```python
from build123d import *

# Parameters (mm, degrees)
CROQUIS1_W                   = 482.6
CROQUIS1_H                   = 634.238
BRIDA_BASE1_DEPTH            = 1.524
CROQUIS6_R                   = 3.9624
CROQUIS6_W                   = 6.35
CROQUIS6_H                   = 3.048
CORTAR_EXTRUIR1_DEPTH        = 399.487732229
BRIDA_START                  = -218.948
BRIDA_DE_ARISTA1_DEPTH       = 437.896
BRIDA_START_2                = -219.1004
BRIDA_DE_ARISTA1_2_OUTLINE_W = 0.1524
BRIDA_DE_ARISTA1_2_OUTLINE_H = 1.524
BRIDA_DE_ARISTA1_2_DEPTH     = 0.1524
BRIDA_START_3                = 218.948
BRIDA_DE_ARISTA1_3_OUTLINE_W = 0.1524
BRIDA_DE_ARISTA1_3_OUTLINE_H = 1.524
BRIDA_DE_ARISTA1_3_DEPTH     = 0.1524
BRIDA_DE_ARISTA1_4_DEPTH     = 437.896
CORTAR_EXTRUIR2_REACH        = 400.806
CROQUIS13_R                  = 3.9624
CROQUIS13_R_2                = 2.8956
CROQUIS13_R_3                = 1.27
CROQUIS13_W                  = 139.7
CROQUIS13_H                  = 124.714


# Read off the part's stored shape, not the designer's step: Brida de arista1
# Sheet-metal steps are written as plain solids
with BuildPart() as part:
    # Croquis1 → Brida base1 (new body)
    with BuildSketch(Plane.XY):
        Rectangle(CROQUIS1_W, CROQUIS1_H)
    extrude(amount=-BRIDA_BASE1_DEPTH)

    # Croquis6 → Cortar-Extruir1 (cut, through all)
    with BuildSketch(Plane.XY):
        with Locations((231.648, 317.627)):
            Circle(CROQUIS6_R)
        with Locations((-231.648, 317.627)):
            Circle(CROQUIS6_R)
        with Locations((-231.648, -317.627)):
            Circle(CROQUIS6_R)
        with Locations((231.648, -317.627)):
            Circle(CROQUIS6_R)
        with Locations((-222.123, 315.595)):
            Rectangle(CROQUIS6_W, CROQUIS6_H)
        with Locations((222.123, 315.595)):
            Rectangle(CROQUIS6_W, CROQUIS6_H)
        with Locations((-222.123, -315.595)):
            Rectangle(CROQUIS6_W, CROQUIS6_H)
        with Locations((222.123, -315.595)):
            Rectangle(CROQUIS6_W, CROQUIS6_H)
    extrude(amount=-CORTAR_EXTRUIR1_DEPTH, mode=Mode.SUBTRACT)

    # Brida de arista1 outline → Brida de arista1 (cut)
    with BuildSketch(Plane.YZ.offset(BRIDA_START)):
        with BuildLine():
            ThreePointArc((-316.710645431, -1.524), (-315.595, -0.408354569), (-314.071, 0))
            Line((-314.071, 0), (-317.119, 0))
            Line((-317.119, 0), (-317.119, -1.524))
            Line((-317.119, -1.524), (-316.710645431, -1.524))
        make_face()
        with BuildLine():
            Line((317.119, 0), (314.071, 0))
            ThreePointArc((314.071, 0), (315.595, -0.408354569), (316.710645431, -1.524))
            Line((316.710645431, -1.524), (317.119, -1.524))
            Line((317.119, -1.524), (317.119, 0))
        make_face()
    extrude(amount=BRIDA_DE_ARISTA1_DEPTH, mode=Mode.SUBTRACT)

    # Brida de arista1 2 outline → Brida de arista1 2 (cut)
    with BuildSketch(Plane.YZ.offset(BRIDA_START_2)):
        with Locations((-313.9948, -0.762)):
            Rectangle(BRIDA_DE_ARISTA1_2_OUTLINE_W, BRIDA_DE_ARISTA1_2_OUTLINE_H)
        with Locations((313.9948, -0.762)):
            Rectangle(BRIDA_DE_ARISTA1_2_OUTLINE_W, BRIDA_DE_ARISTA1_2_OUTLINE_H)
    extrude(amount=BRIDA_DE_ARISTA1_2_DEPTH, mode=Mode.SUBTRACT)

    # Brida de arista1 3 outline → Brida de arista1 3 (cut)
    with BuildSketch(Plane.YZ.offset(BRIDA_START_3)):
        with Locations((-313.9948, -0.762)):
            Rectangle(BRIDA_DE_ARISTA1_3_OUTLINE_W, BRIDA_DE_ARISTA1_3_OUTLINE_H)
        with Locations((313.9948, -0.762)):
            Rectangle(BRIDA_DE_ARISTA1_3_OUTLINE_W, BRIDA_DE_ARISTA1_3_OUTLINE_H)
    extrude(amount=BRIDA_DE_ARISTA1_3_DEPTH, mode=Mode.SUBTRACT)

    # Brida de arista1 4 outline → Brida de arista1 4 (add)
    with BuildSketch(Plane.YZ.offset(BRIDA_START)):
        with BuildLine():
            ThreePointArc((-315.595, -3.048), (-315.148630735, -1.970369265), (-314.071, -1.524))
            Line((-314.071, -1.524), (-316.710645431, -1.524))
            ThreePointArc((-316.710645431, -1.524), (-317.015141918, -2.259119551), (-317.119, -3.048))
            Line((-317.119, -3.048), (-317.119, -16.002))
            Line((-317.119, -16.002), (-315.595, -16.002))
            Line((-315.595, -16.002), (-315.595, -3.048))
        make_face()
        with BuildLine():
            Line((316.710645431, -1.524), (314.071, -1.524))
            ThreePointArc((314.071, -1.524), (315.148630735, -1.970369265), (315.595, -3.048))
            Line((315.595, -3.048), (315.595, -16.002))
            Line((315.595, -16.002), (317.119, -16.002))
            Line((317.119, -16.002), (317.119, -3.048))
            ThreePointArc((317.119, -3.048), (317.015141918, -2.259119551), (316.710645431, -1.524))
        make_face()
    extrude(amount=BRIDA_DE_ARISTA1_4_DEPTH)

    # Croquis13 → Cortar-Extruir2 (cut, up to next)
    with BuildSketch(Plane.XY, mode=Mode.PRIVATE) as cortar_extruir2_sk1:
        with Locations((-231.648, -158.877)):
            Circle(CROQUIS13_R)
    cortar_extruir2_tool1 = extrude(cortar_extruir2_sk1.sketch, amount=-CORTAR_EXTRUIR2_REACH, mode=Mode.PRIVATE) & part.part
    # Croquis13 → Cortar-Extruir2 (cut, up to next)
    with BuildSketch(Plane.XY, mode=Mode.PRIVATE) as cortar_extruir2_sk2:
        with Locations((231.648, 158.877)):
            Circle(CROQUIS13_R)
    cortar_extruir2_tool2 = extrude(cortar_extruir2_sk2.sketch, amount=-CORTAR_EXTRUIR2_REACH, mode=Mode.PRIVATE) & part.part
    # Croquis13 → Cortar-Extruir2 (cut, up to next)
    with BuildSketch(Plane.XY, mode=Mode.PRIVATE) as cortar_extruir2_sk3:
        with Locations((-14.224, 117.983)):
            Circle(CROQUIS13_R_2)
    cortar_extruir2_tool3 = extrude(cortar_extruir2_sk3.sketch, amount=-CORTAR_EXTRUIR2_REACH, mode=Mode.PRIVATE) & part.part
    # Croquis13 → Cortar-Extruir2 (cut, up to next)
    with BuildSketch(Plane.XY, mode=Mode.PRIVATE) as cortar_extruir2_sk4:
        with Locations((63.5, 116.967)):
            Circle(CROQUIS13_R_3)
    cortar_extruir2_tool4 = extrude(cortar_extruir2_sk4.sketch, amount=-CORTAR_EXTRUIR2_REACH, mode=Mode.PRIVATE) & part.part
    # Croquis13 → Cortar-Extruir2 (cut, up to next)
    with BuildSketch(Plane.XY, mode=Mode.PRIVATE) as cortar_extruir2_sk5:
        with Locations((14.478, 117.983)):
            Circle(CROQUIS13_R_2)
    cortar_extruir2_tool5 = extrude(cortar_extruir2_sk5.sketch, amount=-CORTAR_EXTRUIR2_REACH, mode=Mode.PRIVATE) & part.part
    # Croquis13 → Cortar-Extruir2 (cut, up to next)
    with BuildSketch(Plane.XY, mode=Mode.PRIVATE) as cortar_extruir2_sk6:
        with Locations((127, 116.967)):
            Circle(CROQUIS13_R_3)
    cortar_extruir2_tool6 = extrude(cortar_extruir2_sk6.sketch, amount=-CORTAR_EXTRUIR2_REACH, mode=Mode.PRIVATE) & part.part
    # Croquis13 → Cortar-Extruir2 (cut, up to next)
    with BuildSketch(Plane.XY, mode=Mode.PRIVATE) as cortar_extruir2_sk7:
        Rectangle(CROQUIS13_W, CROQUIS13_H)
    cortar_extruir2_tool7 = extrude(cortar_extruir2_sk7.sketch, amount=-CORTAR_EXTRUIR2_REACH, mode=Mode.PRIVATE) & part.part
    add(cortar_extruir2_tool1.solids().sort_by_distance((-231.648, -158.877, 0))[0], mode=Mode.SUBTRACT)
    add(cortar_extruir2_tool2.solids().sort_by_distance((231.648, 158.877, 0))[0], mode=Mode.SUBTRACT)
    add(cortar_extruir2_tool3.solids().sort_by_distance((-14.224, 117.983, 0))[0], mode=Mode.SUBTRACT)
    add(cortar_extruir2_tool4.solids().sort_by_distance((63.5, 116.967, 0))[0], mode=Mode.SUBTRACT)
    add(cortar_extruir2_tool5.solids().sort_by_distance((14.478, 117.983, 0))[0], mode=Mode.SUBTRACT)
    add(cortar_extruir2_tool6.solids().sort_by_distance((127, 116.967, 0))[0], mode=Mode.SUBTRACT)
    add(cortar_extruir2_tool7.solids().sort_by_distance((0, 0, 0))[0], mode=Mode.SUBTRACT)


solid = part.part
```
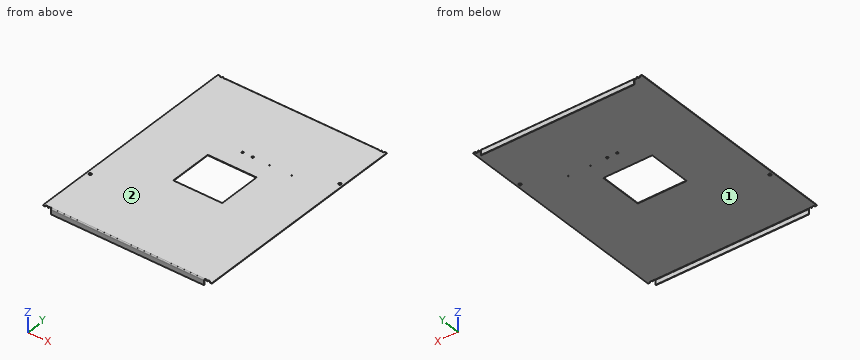
Design review of the part built by this model. Coordinates are the model's own, in mm. Face numbers are marked on the shaded views. Coordinates: 2 decimals unless noted, no trailing zeros. Loops run counter-clockwise (first coordinate to the right, second up) from the corner with the lowest first, then second, coordinate; pieces in that order, holes last.
Q1. We need section C-C on x = -205. State the section outline as (y, z) points (3 decimals).
Reported:
outline: (-317.119, -16.002) - (-315.595, -16.002) - (-315.595, -3.048) arc R1.524 cw to (-314.071, -1.524) - (314.071, -1.524) arc R1.524 cw to (315.595, -3.048) - (315.595, -16.002) - (317.119, -16.002) - (317.119, -3.048) arc R3.048 ccw to (314.071, 0) - (-314.071, 0) arc R3.048 ccw to (-317.119, -3.048) - close
Q2. We need section B-B on z = -9.25. State the section outline as (x, y) points (3 decimals).
Reported:
outline: (-218.948, -317.119) - (218.948, -317.119) - (218.948, -315.595) - (-218.948, -315.595) - close; (-218.948, 315.595) - (218.948, 315.595) - (218.948, 317.119) - (-218.948, 317.119) - close
Q3. To check wall thickness, follow line 1 (Y direction, x = 198, z = -14.75) (3 decimals); line 2 (Y direction, x = -16, z = -1.25); line 3 (Z direction, x = -56, y = -214.5). State the ranges of each line that lie inside material, in increasing order.
Reported:
line 1: y = -317.119 to -315.595, 315.595 to 317.119
line 2: y = -316.53 to -62.36, 62.36 to 115.7, 120.27 to 316.53
line 3: z = -1.52 to 0
Q4. The part is to be moulded in two halves that separate along Y. For the marked faces 1 and 2, say which applies: +Y half, -Y half, draft (parallel to the pull), parting line (faces both ways), or undercut.
Reported:
face 1: undercut
face 2: draft
Q5. For pin 1 (0.8 mm diameter, centred on x = 16.5, z = -0.5, fed in from +Y); pin 2 (1.6 mm diameter, centred on y = 315.5, z = -11.5, fed in from -X); pin 3 (6.5 mm diameter, centred on x = 14.478, y = 117.983, fed in from +Z); pin 4 (1.6 mm diameter, centred on y = 315, z = -5, fed in from +X), all flat-tipped, find the tip position at first contact; note any pin that passes through.
Reported:
pin 1: stops at y = 316.23
pin 2: stops at x = -218.95
pin 3: stops at z = 0
pin 4: stops at x = 218.95
Q6. We need section D-D on y = -69.5. State the section outline as (x, z) points, and give its area (3 significant figures).
Reported:
outline: (-241.3, -1.52) - (241.3, -1.52) - (241.3, 0) - (-241.3, 0) - close
area: 735 mm2
Q7. We need section A-A on x = -56. State the section outline as (y, z) points (3 decimals).
Reported:
outline: (-317.119, -16.002) - (-315.595, -16.002) - (-315.595, -3.048) arc R1.524 cw to (-314.071, -1.524) - (-62.357, -1.524) - (-62.357, 0) - (-314.071, 0) arc R3.048 ccw to (-317.119, -3.048) - close; (62.357, -1.524) - (314.071, -1.524) arc R1.524 cw to (315.595, -3.048) - (315.595, -16.002) - (317.119, -16.002) - (317.119, -3.048) arc R3.048 ccw to (314.071, 0) - (62.357, 0) - close
